Autodesk Inventor part; units mm, degrees
ref_plane "YZ Plane" through (0, 0, 0) normal (1, 0, 0) x (0, 1, 0)
ref_plane "XZ Plane" through (0, 0, 0) normal (0, 1, 0) x (-1, 0, 0)
ref_plane "XY Plane" through (0, 0, 0) normal (0, 0, 1) x (1, 0, 0)
sketch "Sketch1" plane through (0, 0, 0) normal (0, 0, 1) x (1, 0, 0)
  line L0 (88.9, -44.45) -> (-88.9, -44.45)
  line L1 (-88.9, -44.45) -> (-88.9, 44.45)
  line L2 (-88.9, 44.45) -> (88.9, 44.45)
  line L3 (88.9, 44.45) -> (88.9, -44.45)
  line L4 (88.9, -44.45) -> (-88.9, 44.45) construction
  line L5 (-88.9, -44.45) -> (88.9, 44.45) construction
  line L6 (-38.735, -25.4) -> (-76.2, -25.4)
  line L7 (-76.2, -25.4) -> (-76.2, 25.4)
  line L8 (-76.2, 25.4) -> (-38.735, 25.4)
  line L9 (-38.735, 25.4) -> (-38.735, -25.4)
  line L10 (-38.735, -25.4) -> (-76.2, 25.4) construction
  line L11 (-76.2, -25.4) -> (-38.735, 25.4) construction
  line L12 (18.7325, -25.4) -> (-18.7325, -25.4)
  line L13 (-18.7325, -25.4) -> (-18.7325, 25.4)
  line L14 (-18.7325, 25.4) -> (18.7325, 25.4)
  line L15 (18.7325, 25.4) -> (18.7325, -25.4)
  line L16 (18.7325, -25.4) -> (-18.7325, 25.4) construction
  line L17 (-18.7325, -25.4) -> (18.7325, 25.4) construction
  line L18 (76.2, -25.4) -> (38.735, -25.4)
  line L19 (38.735, -25.4) -> (38.735, 25.4)
  line L20 (38.735, 25.4) -> (76.2, 25.4)
  line L21 (76.2, 25.4) -> (76.2, -25.4)
  line L22 (76.2, -25.4) -> (38.735, 25.4) construction
  line L23 (38.735, -25.4) -> (76.2, 25.4) construction
  line L24 (-38.735, 25.4) -> (-38.735, -25.4)
  line L25 (-38.735, -25.4) -> (-18.7325, -25.4)
  line L26 (-18.7325, -25.4) -> (-18.7325, 25.4)
  line L27 (-18.7325, 25.4) -> (-38.735, 25.4)
  line L28 (18.7325, 25.4) -> (18.7325, -25.4)
  line L29 (18.7325, -25.4) -> (38.735, -25.4)
  line L30 (38.735, -25.4) -> (38.735, 25.4)
  line L31 (38.735, 25.4) -> (18.7325, 25.4)
  line L32 (-76.2, -25.4) -> (76.2, -25.4)
  line L33 (76.2, -25.4) -> (76.2, -38.1)
  line L34 (76.2, -38.1) -> (-76.2, -38.1)
  line L35 (-76.2, -38.1) -> (-76.2, -25.4)
  point P0 (0, 0)
  point P1 (-57.4675, 0)
  point P2 (-57.4675, 0)
  point P3 (0, 0)
  point P4 (57.4675, 0)
  point P5 (0, 0)
  point P6 (57.4675, 0)
  dimension "d0" = 177.8
  dimension "d1" = 88.9
  dimension "d2" = 37.465
  dimension "d3" = 50.8
  dimension "d4" = 12.7
  dimension "d5" = 12.7
  dimension "d6" = 12.7
extrude "Extrusion1" add sketch "Sketch1" along normal blind 17.78
extrude "Extrusion2" add sketch "Sketch1" against normal blind 3.175 contours L0 L1 L2 L3 | L25 L12 L29 L18 L33 L34 L35 L6 | L6 L7 L8 L9 | L9 L27 L13 L25 | L13 L14 L15 L12 | L15 L31 L19 L29 | L19 L20 L21 L18
extrude "Extrusion3" add sketch "Sketch1" along normal blind 6.35 contours L25 L12 L29 L18 L33 L34 L35 L6 | L9 L27 L13 L25 | L15 L31 L19 L29
sketch "Sketch2" plane through (0, 0, 17.78) normal (0, 0, 1) x (1, 0, 0)
  line L0 (-38.735, -25.4) -> (-76.2, -25.4)
  line L1 (-38.735, -25.4) -> (-38.735, -44.45)
  line L2 (88.9, -44.45) -> (-88.9, -44.45)
  line L3 (-38.735, -44.45) -> (-45.085, -44.45)
  line L4 (76.2, -38.1) -> (-76.2, -38.1)
  line L5 (-45.085, -38.1) -> (-45.085, -44.45)
  line L6 (-45.085, -38.1) -> (-38.735, -38.1)
  point P0 (0, 0)
  dimension "d13" = 6.35
extrude "Extrusion4" cut sketch "Sketch2" against normal up to surface (11.43 mm away)
pattern_linear "Rectangular Pattern1" count 3 spacing 57.15 along (1, 0, 0) of "Extrusion4"
equation "\"d5\" = d4"
The listing builds one solid part. Answer for the finished solid, in the listing's coordinates (mm). A direction names the side the tool comes from. Coordinates: 2 decimals unless noted, no trailing zeros. Loops run counter-clockwise (first coordinate to the right, second up) from the corner with the lowest first, then second, coordinate; pieces in that order, holes last.
1) Find section A-A on z = 13.5. Write down the section's boundary in (x, y) (3 decimals), then the cut area to 3 significant figures.
2) Find section C-C on z = 2. Give the number of separate pieces and of enclosed holes in the cut face, then the cut area to 3 significant figures.
3) Determine the mould class of faces 4 (the face through (18.732, 0, 3)), 5 (the face through (1, -44.45, 7)), 6 (the face through (12.065, -41, 12)) for opening direction Y: pulls with the +Y half, pulls with the -Y half, needs draft (parallel to the pull), parting line crosses it, or undercut.
4) Find section B-B on y = -32.5. Write down the section's boundary in (x, z) (3 decimals), then the cut area to 3 significant figures.
5) A tool of negligible diameter and unlimited length cuts with its end or side. For faces 1 (the face through (88.9, 1, 7)), 2 (the face through (18.415, -41, 12)), 3 (the face through (76.2, -6, 9)), from which of +Z, -Z, +X, -X, +Y, -Y can it reach the whole face along a straight path? Write none if from no direction.
6) Flat-ended cylindrical pins translate along their axes: pin 1 Ø18.5 at (x, y) = (52.5, -4.5) entering from +Z; pin 2 Ø6 at (x, y) = (16.5, -6) entering from +Z. Find the tip coordinate at first contact, or state that the pin passes through.
7) Find section D-D on x = 35. Write down the section's boundary in (y, z) (3 decimals).
8) Find the intervals of material crossed by L1, parallel to X at y = 3, z = 5 (1 decimal); L2, parallel to Y at x = -48.5, z = 3.25; L3, parallel to Y at x = -11.5, z = 13.25, in increasing order.
Values:
1. outline: (-88.9, -44.45) - (-45.085, -44.45) - (-45.085, -38.1) - (-76.2, -38.1) - (-76.2, 25.4) - (76.2, 25.4) - (76.2, -38.1) - (75.565, -38.1) - (75.565, -44.45) - (88.9, -44.45) - (88.9, 44.45) - (-88.9, 44.45) - close; (-38.735, -44.45) - (12.065, -44.45) - (12.065, -38.1) - (-38.735, -38.1) - close; (18.415, -44.45) - (69.215, -44.45) - (69.215, -38.1) - (18.415, -38.1) - close
1. area: 6,010 mm2
2. separate pieces: 1
2. enclosed holes: 3
2. area: 10,100 mm2
3. face 4: undercut
3. face 5: pulls with the -Y half
3. face 6: needs draft
4. outline: (-88.9, -3.175) - (88.9, -3.175) - (88.9, 17.78) - (76.2, 17.78) - (76.2, 6.35) - (-76.2, 6.35) - (-76.2, 17.78) - (-88.9, 17.78) - close
4. area: 1,980 mm2
5. face 1: +Z, -Z, +X, +Y, -Y
5. face 2: +Z, -Y
5. face 3: +Z
6. pin 1: stops at z = 0
6. pin 2: stops at z = 6.35
7. outline: (-44.45, -3.175) - (44.45, -3.175) - (44.45, 17.78) - (25.4, 17.78) - (25.4, 6.35) - (-38.1, 6.35) - (-38.1, 17.78) - (-44.45, 17.78) - close
8. L1: x = -88.9 to -76.2, -38.7 to -18.7, 18.7 to 38.7, 76.2 to 88.9
8. L2: y = -44.45 to -25.4, 25.4 to 44.45
8. L3: y = -44.45 to -38.1, 25.4 to 44.45
